Design review of the part built by this model. Coordinates are the model's own, in mm. Coordinates: 2 decimals unless noted, no trailing zeros. Loops run counter-clockwise (first coordinate to the right, second up) from the corner with the lowest first, then second, coordinate; pieces in that order, holes last. Notation, with made-up numbers: (-26.75, -33.5) -> (27.25, -33.5) arc R27 cw to (27.25, -8.5) -> close; hole circle Ø4 at (54.5, 23.25). An arc over 180 degrees is marked (long way). Use one line per item in the form item = value. Start each with the question number.
1. For pin 1 (2 mm diameter, centred on y = 39, z = 1, fed in from +X), flat-tipped, find the tip position at first contact; note if it passes through.
2. Consider section B-B (z = 2.95). State the section outline as (x, y) points, then the cut area to 3 significant figures.
3. The part is to be moulded in two halves that separate along X. For faces 1 (the face through (126.548, 195.935, 1.972)), 2 (the face through (78.94, 45.67, 1.97)), 3 (the face through (59, 72, 4)), say which applies: released by +X, released by -X, zero draft, split by the parting line, or undercut.
4. Consider section D-D (y = 118). State the section outline as (x, z) points.
5. Wall thickness on line 1 (Y direction, x = 130, z = 2.2); line 2 (Y direction, x = 110, z = 0.4); line 3 (X direction, y = -29.5, z = 1.25): over which ranges is each line inside the solid? List them lowest first. Write a range as from..to.
6. Consider section C-C (x = 69). State the section outline as (y, z) points, then the cut area to 3 significant figures.
7. Consider section A-A (x = 113.5). State the section outline as (y, z) points, then the cut area to 3 significant figures.
from build123d import *

# Parameters (mm, degrees)
SKETCH1_R           = 4
BOSS_EXTRUDE1_DEPTH = 4


with BuildPart() as part:
    # Sketch1 → Boss-Extrude1 (new body)
    with BuildSketch(Plane.XY):
        with BuildLine():
            Line((0, 0), (0, -40))
            Line((0, -40), (40, -40))
            Line((40, -40), (118.991479096, 133.781254012))
            ThreePointArc((118.991479096, 133.781254012), (106.386366554, 167.394887458), (140, 180))
            Line((140, 180), (140, 200))
            Line((140, 200), (100, 200))
            Line((100, 200), (0, 0))
        make_face()
        with Locations((129.495739548, 193.231222879)):
            Circle(SKETCH1_R, mode=Mode.SUBTRACT)
    extrude(amount=BOSS_EXTRUDE1_DEPTH)


solid = part.part
Geometry check:
q1.pin_1 = 76.36
q2.outline = (0, -40) -> (40, -40) -> (118.99, 133.78) arc R25.38 cw to (140, 180) -> (140, 200) -> (100, 200) -> (0, 0) -> close; hole circle Ø8 at (129.5, 193.23)
q2.area = 11,500 mm²
q3.face_1 = undercut
q3.face_2 = released by +X
q3.face_3 = zero draft
q4.outline = (59, 0) -> (111.82, 0) -> (111.82, 4) -> (59, 4) -> close
q5.line_1 = 182.27..189.26, 197.2..200
q5.line_2 = 114..140.63, 173.15..200
q5.line_3 = 0..44.77
q6.outline = (23.8, 0) -> (138, 0) -> (138, 4) -> (23.8, 4) -> close
q6.area = 457 mm²
q7.outline = (121.7, 0) -> (137.18, 0) -> (137.18, 4) -> (121.7, 4) -> close; (176.6, 0) -> (200, 0) -> (200, 4) -> (176.6, 4) -> close
q7.area = 156 mm²
